Autodesk Inventor part; units mm, degrees
ref_plane "YZ Plane" through (0, 0, 0) normal (1, 0, 0) x (0, 1, 0)
ref_plane "XZ Plane" through (0, 0, 0) normal (0, 1, 0) x (-1, 0, 0)
ref_plane "XY Plane" through (0, 0, 0) normal (0, 0, 1) x (1, 0, 0)
sketch "Sketch1" plane through (0, 0, 0) normal (0, 0, 1) x (1, 0, 0)
  line L0 (0, 0) -> (160, 0)
  line L1 (160, 0) -> (118.589, -154.5481) construction
  line L2 (0, 0) -> (41.411, -154.5481) construction
  line L3 (41.411, -154.5481) -> (118.589, -154.5481)
  circle A0 centre (235.8871, -103.156) radius 80 construction
  line L4 (160, 0) -> (256.5926, -25.8819)
  line L5 (118.589, -154.5481) -> (215.1815, -180.43)
  arc A1 (215.1815, -180.43) -> (256.5926, -25.8819) centre (235.8871, -103.156) ccw
  circle A2 centre (-75.8871, -103.156) radius 80 construction
  line L6 (0, 0) -> (-96.5926, -25.8819)
  line L7 (41.411, -154.5481) -> (-55.1815, -180.43)
  arc A3 (-96.5926, -25.8819) -> (-55.1815, -180.43) centre (-75.8871, -103.156) ccw
  dimension "d0" = 160
  dimension "d1" = 160
  dimension "d2" = 160
  dimension "d3" = 75
  dimension "d4" = 75
  dimension "d5" = 160
  dimension "d6" = 100
  dimension "d7" = 160
  dimension "d9" = 100
extrude "Extrusion1" add sketch "Sketch1" along normal blind 41.5
sketch "Sketch2" plane through (0, 0, 41.5) normal (0, 0, 1) x (1, 0, 0)
  line L0 (-26.5, -133) -> (186.5, -133)
  line L1 (186.5, -133) -> (186.5, -20)
  line L2 (186.5, -20) -> (-26.5, -20)
  line L3 (-26.5, -20) -> (-26.5, -133)
  line L4 (160, 0) -> (0, 0)
  point P0 (80, -20)
  point P1 (80, 0)
  dimension "d12" = 213
  dimension "d13" = 113
  dimension "d14" = 20
extrude "Extrusion2" cut sketch "Sketch2" against normal through all
sketch "Sketch3" plane through (0, 0, 41.5) normal (0, 0, 1) x (1, 0, 0)
  line L0 (-26.5, -133) -> (-26.5, -20) construction
  line L1 (-26.5, -20) -> (186.5, -20) construction
  line L2 (186.5, -20) -> (186.5, -133) construction
  line L3 (186.5, -133) -> (-26.5, -133) construction
  line L4 (-48.0481, 1.5481) -> (-48.0481, -154.5481) construction
  line L5 (-48.0481, -154.5481) -> (208.0481, -154.5481) construction
  line L6 (208.0481, -154.5481) -> (208.0481, 1.5481) construction
  line L7 (208.0481, 1.5481) -> (-48.0481, 1.5481) construction
  line L8 (41.411, -154.5481) -> (118.589, -154.5481) construction
  line L9 (-48.0481, 1.5481) -> (-48.0481, -178.5186) construction
  line L10 (-55.1815, -180.43) -> (41.411, -154.5481) construction
  line L11 (208.0481, 1.5481) -> (208.0481, -178.5186) construction
  line L12 (118.589, -154.5481) -> (215.1815, -180.43) construction
  line L13 (-48.0481, -178.5186) -> (208.0481, -178.5186) construction
  line L14 (-48.0481, 1.5481) -> (208.0481, 1.5481) construction
  line L15 (160, 0) -> (256.5926, -25.8819) construction
  line L16 (208.2963, -12.941) -> (208.0481, -178.5186)
  line L17 (208.2963, -12.941) -> (256.5926, -25.8819)
  line L18 (208.0481, -178.5186) -> (215.1815, -180.43)
  arc A0 (215.1815, -180.43) -> (256.5926, -25.8819) centre (235.8871, -103.156) ccw
  line L19 (208.0481, 1.5481) -> (-166.9519, 1.5481)
  line L20 (-166.9519, 1.5481) -> (-166.9519, -188.4519)
  line L21 (-166.9519, -188.4519) -> (208.0481, -188.4519)
  line L22 (208.0481, -188.4519) -> (208.0481, 1.5481)
  point P0 (0, 0)
  point P1 (80, -154.5481)
  dimension "d17" = 190
  dimension "d18" = 375
extrude "Extrusion3" cut sketch "Sketch3" against normal through all contours L22 L21 L20 L19
sketch "Sketch4" plane through (0, 0, 41.5) normal (0, 0, 1) x (1, 0, 0)
  arc A0 (215.1815, -180.43) -> (256.5926, -25.8819) centre (235.8871, -103.156) ccw
  circle A1 centre (235.8871, -103.156) radius 7
  point P0 (0, 0)
  dimension "d21" = 14
extrude "Extrusion4" cut sketch "Sketch4" against normal through all
sketch "Sketch5" plane through (208.0481, -178.5186, 41.5) normal (-1, 0, 0) x (0, 0, 1)
  line L0 (-41.5, 165.6442) -> (0, 165.6442)
  line L1 (-41.5, 0) -> (-41.5, 165.6442)
  line L2 (0, 0) -> (-41.5, 0)
  line L3 (0, 165.6442) -> (0, 0)
  line L4 (-33, 157.1442) -> (-8.5, 157.1442)
  line L5 (-8.5, 157.1442) -> (-8.5, 8.5)
  line L6 (-8.5, 8.5) -> (-33, 8.5)
  line L7 (-33, 8.5) -> (-33, 157.1442)
  point P0 (-41.5, 178.5186)
  dimension "d24" = 8.5
extrude "Extrusion5" add sketch "Sketch5" along normal blind 13 contours L4 L5 L6 L7
sketch "Sketch6" plane through (208.0481, -170.0186, 8.5) normal (0, 0, -1) x (-1, 0, 0)
  circle A0 centre (8, 74.3221) radius 2.5
  line L0 (0, -8.5) -> (0, 157.1442)
  point P0 (208.0481, 170.0186)
  point P1 (0, 74.3221)
  dimension "d27" = 5
  dimension "d28" = 8
extrude "Extrusion6" cut sketch "Sketch6" against normal through all
sketch "Sketch7" plane through (0, 0, 0) normal (0, 0, -1) x (-1, 0, 0)
  circle A0 centre (-235.8871, -103.156) radius 7
  line L0 (-208.0481, -178.5186) -> (-208.0481, -12.8745)
  line L1 (-208.0481, -12.8745) -> (-256.5926, -25.8819)
  arc A1 (-256.5926, -25.8819) -> (-215.1815, -180.43) centre (-235.8871, -103.156) ccw
  line L2 (-215.1815, -180.43) -> (-208.0481, -178.5186)
  line L3 (-254.522, -33.6093) -> (-216.0481, -23.3003)
  line L4 (-216.0481, -23.3003) -> (-216.0481, -172.38)
  line L5 (-216.0481, -172.38) -> (-217.2521, -172.7026)
  arc A2 (-254.522, -33.6093) -> (-217.2521, -172.7026) centre (-235.8871, -103.156) ccw
  circle A3 centre (-235.8871, -103.156) radius 15
  point P0 (0, 0)
  dimension "d31" = 8
  dimension "d32" = 8
extrude "Extrusion7" cut sketch "Sketch7" against normal through all contours L3 L4 L5 A2
sketch "Sketch8" plane through (0, 0, 0) normal (0, 0, -1) x (-1, 0, 0)
  circle A0 centre (-235.8871, -103.156) radius 7 construction
  circle A1 centre (-235.8871, -103.156) radius 15 construction
  line L0 (-235.8871, -103.156) -> (-159.7277, -103.156) construction
  line L1 (-221.7449, -98.156) -> (-123.6167, -98.156) construction
  line L2 (-221.7449, -108.156) -> (-123.6167, -108.156) construction
  line L3 (-233.1461, -88.4085) -> (-184.082, -3.427) construction
  line L4 (-224.4859, -93.4085) -> (-175.4217, -8.427) construction
  line L5 (-247.2883, -93.4085) -> (-296.3524, -8.427) construction
  line L6 (-238.628, -88.4085) -> (-287.6921, -3.427) construction
  line L7 (-250.0292, -108.156) -> (-348.1575, -108.156) construction
  line L8 (-250.0292, -98.156) -> (-348.1575, -98.156) construction
  line L9 (-238.628, -117.9034) -> (-287.6921, -202.885) construction
  line L10 (-247.2883, -112.9034) -> (-296.3524, -197.885) construction
  line L11 (-224.4859, -112.9034) -> (-175.4217, -197.885) construction
  line L12 (-233.1461, -117.9034) -> (-184.082, -202.885) construction
  line L13 (-216.0481, -23.3003) -> (-216.0481, -172.38) construction
  arc A2 (-254.522, -33.6093) -> (-217.2521, -172.7026) centre (-235.8871, -103.156) ccw construction
  line L14 (-254.522, -33.6093) -> (-216.0481, -23.3003) construction
  line L15 (-216.0481, -172.38) -> (-217.2521, -172.7026) construction
  line L16 (-221.7449, -98.156) -> (-216.0481, -98.156)
  line L17 (-221.7449, -108.156) -> (-216.0481, -108.156)
  line L18 (-224.4859, -112.9034) -> (-216.0481, -127.518)
  line L19 (-233.1461, -117.9034) -> (-216.0481, -147.518)
  line L20 (-238.628, -117.9034) -> (-267.47, -167.8593)
  line L21 (-276.1303, -162.8593) -> (-247.2883, -112.9034)
  line L22 (-250.0292, -108.156) -> (-307.7132, -108.156)
  line L23 (-250.0292, -98.156) -> (-307.7132, -98.156)
  line L24 (-247.2883, -93.4085) -> (-276.1303, -43.4527)
  line L25 (-238.628, -88.4085) -> (-267.47, -38.4527)
  line L26 (-233.1461, -88.4085) -> (-216.0481, -58.7939)
  line L27 (-224.4859, -93.4085) -> (-216.0481, -78.7939)
  line L28 (-216.0481, -58.7939) -> (-216.0481, -78.7939)
  line L29 (-216.0481, -98.156) -> (-216.0481, -108.156)
  line L30 (-216.0481, -127.518) -> (-216.0481, -147.518)
  arc A3 (-267.47, -38.4527) -> (-276.1303, -43.4527) centre (-235.8871, -103.156) ccw
  arc A4 (-307.7132, -98.156) -> (-307.7132, -108.156) centre (-235.8871, -103.156) ccw
  arc A5 (-276.1303, -162.8593) -> (-267.47, -167.8593) centre (-235.8871, -103.156) ccw
  arc A6 (-221.7449, -108.156) -> (-221.7449, -98.156) centre (-235.8871, -103.156) ccw
  arc A7 (-233.1461, -117.9034) -> (-224.4859, -112.9034) centre (-235.8871, -103.156) ccw
  arc A8 (-247.2883, -112.9034) -> (-238.628, -117.9034) centre (-235.8871, -103.156) ccw
  arc A9 (-250.0292, -98.156) -> (-250.0292, -108.156) centre (-235.8871, -103.156) ccw
  arc A10 (-238.628, -88.4085) -> (-247.2883, -93.4085) centre (-235.8871, -103.156) ccw
  arc A11 (-224.4859, -93.4085) -> (-233.1461, -88.4085) centre (-235.8871, -103.156) ccw
  point P0 (0, 0)
  dimension "d36" = 5
  dimension "d37" = 5
  dimension "d40" = 360
extrude "Extrusion8" add sketch "Sketch8" against normal blind 41.5
properties part number "Riser Base" material "ABS Plastic"
Model file for the job. Use its own axes, mm. A direction names the side the tool comes from. Round coordinates to 2 decimals unless told otherwise and drop trailing zeros. Order: outer loops, then holes, each group sorted by start corner. A loop starts at its lowest first (then second) coordinate and runs counter-clockwise, first axis right, second up.
(1) Band-saw the part on B-B (x = 241). List the corners of the cut face in (y, z), then the cut area to 3 significant figures.
(2) Band-saw the part on A-A (y = -53). List the corners of the cut face in (x, z).
(3) Drill centre lines: line 1 (X direction, y = -54.5, z = 26); line 2 (X direction, y = -131, z = 2.5); line 3 (Y direction, x = 296, z = 22). Where is each one in solid material? Low to high.
(4) Pin check, flat tips, straight feed: pin 1 (12.5 mm diameter, centred on y = -158, z = 16, fed in from +X); pin 2 (3 mm diameter, centred on x = 200.05, y = -95.7, fed in from -Z); pin 3 (6.5 mm diameter, centred on x = 203, z = 17.5, fed in from -Y); pin 4 (10.5 mm diameter, centred on y = -33, z = 27.5, fed in from +X). Stop position of each tip, or through.
(5) Band-saw the part on D-D (x = 280.5). List the corners of the cut face in (y, z).
(6) Pull direction Y, two halves, no side cores. Call faces 1 (the face through (202, -21.374, 21)), 2 (the face through (250, -104, 0)), 3 (the face through (216.048, -41, 20)): released by +Y, released by -Y, zero draft, split by the parting line, or undercut.
(7) 3-axis set-ups, long thin cutter, end or side, ignore diameter. For faces 4 (the face through (195.048, -95, 21)), 5 (the face through (235.848, -88.156, 20.46)), 6 (the face through (202, -170.019, 21)): which of +Z, -Z, +X, -X, +Y, -Y reach the whole face in a straight line?
(8) Band-saw the part on C-C (x = 259). List the corners of the cut face in (y, z).
Verdict:
1. outline: (-182.99, 0) - (-174.97, 0) - (-174.97, 41.5) - (-182.99, 41.5) - close; (-122.01, 0) - (-107.94, 0) - (-107.94, 41.5) - (-122.01, 41.5) - close; (-98.37, 0) - (-84.3, 0) - (-84.3, 41.5) - (-98.37, 41.5) - close; (-29.99, 0) - (-21.7, 0) - (-21.7, 41.5) - (-29.99, 41.5) - close
1. area: 1,840 mm2
2. outline: (195.05, 8.5) - (208.05, 8.5) - (208.05, 0) - (216.05, 0) - (216.05, 41.5) - (208.05, 41.5) - (208.05, 33) - (195.05, 33) - close; (259.07, 0) - (270.62, 0) - (270.62, 41.5) - (259.07, 41.5) - close; (287.54, 0) - (298.21, 0) - (298.21, 41.5) - (287.54, 41.5) - close
3. line 1: x = 195.05 to 216.05, 258.21 to 269.75, 288.96 to 299.39
3. line 2: x = 208.05 to 225.58, 246.19 to 257.74, 302.29 to 310.89
3. line 3: y = -155.94 to -142.78, -108.16 to -98.16, -63.53 to -50.37
4. pin 1: stops at x = 299.44
4. pin 2: passes through
4. pin 3: stops at y = -170.02
4. pin 4: stops at x = 282.65
5. outline: (-169.56, 0) - (-159.67, 0) - (-159.67, 41.5) - (-169.56, 41.5) - close; (-108.16, 0) - (-98.16, 0) - (-98.16, 41.5) - (-108.16, 41.5) - close; (-46.64, 0) - (-36.75, 0) - (-36.75, 41.5) - (-46.64, 41.5) - close
6. face 1: released by +Y
6. face 2: zero draft
6. face 3: undercut
7. face 4: +Z, -Z, -X, +Y, -Y
7. face 5: +Z, -Z
7. face 6: +Z, -Z, -X, -Y
8. outline: (-179.74, 0) - (-171.35, 0) - (-171.35, 41.5) - (-179.74, 41.5) - close; (-153.19, 0) - (-133.19, 0) - (-133.19, 41.5) - (-153.19, 41.5) - close; (-108.16, 0) - (-98.16, 0) - (-98.16, 41.5) - (-108.16, 41.5) - close; (-73.12, 0) - (-53.12, 0) - (-53.12, 41.5) - (-73.12, 41.5) - close; (-34.97, 0) - (-26.57, 0) - (-26.57, 41.5) - (-34.97, 41.5) - close
